from build123d import *

# Parameters (mm, degrees)
SKETCH_1_R      = 5
EXTRUDE_1_DEPTH = 80
CHAMFER_1_SIZE  = 0.5
SKETCH_2_W      = 2.220028262
SKETCH_2_H      = 1.1


with BuildPart() as part:
    # 草图1 → 拉伸1 (new body)
    with BuildSketch(Plane.XY):
        Circle(SKETCH_1_R)
    extrude(amount=EXTRUDE_1_DEPTH)

    # 倒角1
    chamfer_1_edges = [part.edges().sort_by_distance(p)[0] for p in [
        (-5, 0, 0),
        (-5, 0, 80),
    ]]
    chamfer(chamfer_1_edges, length=CHAMFER_1_SIZE)

    # 草图2 → 切除-旋转1 (revolve, cut)
    with BuildSketch(Plane(origin=(0, 0, 0), x_dir=(1, 0, 0), z_dir=(0, 1, 0))):
        with Locations((5.760014131, -51.839999917)):
            Rectangle(SKETCH_2_W, SKETCH_2_H)
    revolve(axis=Axis((0, 0, 80), (0, 0, -1)), mode=Mode.SUBTRACT)


solid = part.part
For this review, take the finished solid that the model builds, in its own axes (mm). Round coordinates to 2 decimals unless told otherwise and drop trailing zeros. Order: outer loops, then holes, each group sorted by start corner. A loop starts at its lowest first (then second) coordinate and runs counter-clockwise, first axis right, second up. Notation, with made-up numbers: (-17, 23.25) -> (42, 23.25) arc R30 ccw to (42, 46.25) -> close; hole circle Ø2 at (81.5, 66.5). An arc over 180 degrees is marked (long way). Write item = value, one per line. Start each with the question number.
1) Take a section at A-A on z = 7. State the section outline as (x, y) points.
2) Insertion check: pin 1 (4 mm diameter, centred on y = -4, z = 62, fed in from -X); pin 2 (5 mm diameter, centred on y = -2.5, z = 36.5, fed in from -X); pin 3 (2 mm diameter, centred on y = 2.5, z = 26, fed in from +X). Each pin has a flat end and moves straight along its axis. Give the tip position at first contact, or say it passes through.
3) To check wall thickness, follow line 1 (Y direction, x = -0.25, z = 64); line 2 (Z direction, x = -3.5, y = -3.25); line 3 (X direction, y = 0.5, z = 39). State the ranges of each line that lie inside material, in increasing order. Write a range as from..to.
4) The part is to be moulded in two halves that separate along Z. For faces 1 (the face through (2.5, -3.92, 51.83)), 2 (the face through (0, 0, 0)), 3 (the face through (-1.08, -4.88, 65.76)), say which applies: +Z half, -Z half, draft (parallel to the pull), parting line (faces both ways), or undercut.
Verdict:
q1.outline = circle Ø10 at (0, 0)
q2.pin_1 = -4.58
q2.pin_2 = -5
q2.pin_3 = 4.77
q3.line_1 = -4.99..4.99
q3.line_2 = 0.28..51.29, 52.39..79.72
q3.line_3 = -4.97..4.97
q4.face_1 = undercut
q4.face_2 = -Z half
q4.face_3 = draft
